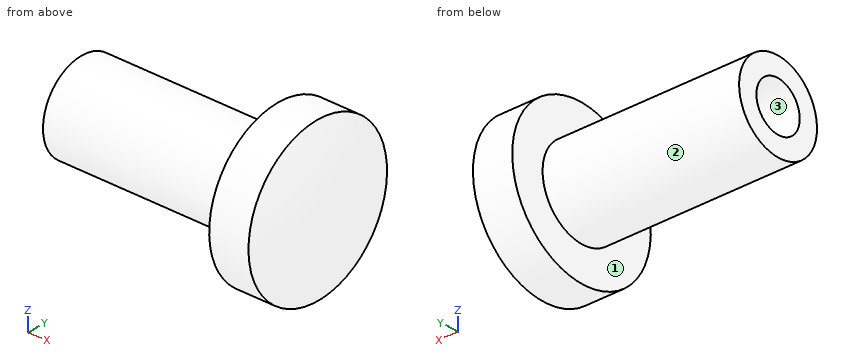
```python
from build123d import *

# Parameters (mm, degrees)
SKETCH2_R          = 1.25
CUT_EXTRUDE1_DEPTH = 11.25
SKETCH3_R          = 1.7
CUT_EXTRUDE2_DEPTH = 0.35


with BuildPart() as part:
    # Sketch1 → Revolve1 (revolve)
    with BuildSketch(Plane.XY, mode=Mode.PRIVATE) as revolve1_sk:
        with BuildLine():
            Line((0, 0), (0, 2.25))
            Line((0, 2.25), (10, 2.25))
            Line((10, 2.25), (10, 4))
            Line((10, 4), (12, 4))
            ThreePointArc((12, 4), (12.635153756, 2.044657673), (12.85, 0))
            Line((12.85, 0), (0, 0))
        make_face()
    revolve(revolve1_sk.sketch.rotate(Axis((0, 0, 0), (1, 0, 0)), 90), axis=Axis((0, 0, 0), (1, 0, 0)))

    # Sketch2 → Cut-Extrude1 (cut)
    with BuildSketch(Plane.ZY):
        Circle(SKETCH2_R)
    extrude(amount=-CUT_EXTRUDE1_DEPTH, mode=Mode.SUBTRACT)

    # Sketch3 → Cut-Extrude2 (cut)
    with BuildSketch(Plane.ZY.offset(-11.25)):
        Circle(SKETCH3_R)
    extrude(amount=-CUT_EXTRUDE2_DEPTH, mode=Mode.SUBTRACT)


solid = part.part
```
Here's how the part is built. I have some questions about the finished solid (model axes, mm). Face numbers are marked on the shaded views. Coordinates: 2 decimals unless noted, no trailing zeros. Order: outer loops, then holes, each group sorted by start corner. A loop starts at its lowest first (then second) coordinate and runs counter-clockwise, first axis right, second up.
1) I need wall thicknesses on line 1 (Y direction, x = 4.25, z = 0); line 2 (Y direction, x = 11.45, z = 0); line 3 (Z direction, x = 0.75, y = 0.25). Which ranges of each line are inside material? Lowest first, please.
2) Imagine slicing it at B-B on y = 0. List the corners of the cut face in (x, z) for me.
3) We'd pull the mould along Z, two halves only. Please class the marked faces 1, 2 and 3: +Z half, -Z half, draft (parallel to the pull), parting line (faces both ways), or undercut.
4) Will these pins go through, and if not, where does the flat tip stop? pin 1 (1 mm diameter, centred on y = 0.5, z = -0.5, fed in from -X); pin 2 (1 mm diameter, centred on y = 0.5, z = 0.5, fed in from +X); pin 3 (2 mm diameter, centred on x = 4, z = -0.5, fed in from +Y).
5) Imagine slicing it at A-A on x = 4.25. List the corners of the cut face in (y, z) for me.
6) Imagine slicing it at D-D on x = 10.5. List the corners of the cut face in (y, z) for me, and give its area (3 significant figures).
Response values:
1. line 1: y = -2.25 to -1.25, 1.25 to 2.25
1. line 2: y = -4 to -1.7, 1.7 to 4
1. line 3: z = -2.24 to -1.22, 1.22 to 2.24
2. outline: (0, -2.25) - (10, -2.25) - (10, -4) - (12, -4) arc R9.84 ccw to (12, 4) - (10, 4) - (10, 2.25) - (0, 2.25) - (0, 1.25) - (11.25, 1.25) - (11.25, 1.7) - (11.6, 1.7) - (11.6, -1.7) - (11.25, -1.7) - (11.25, -1.25) - (0, -1.25) - close
3. face 1: draft
3. face 2: parting line
3. face 3: undercut
4. pin 1: stops at x = 11.6
4. pin 2: stops at x = 12.85
4. pin 3: stops at y = 2.25
5. outline: circle Ø4.5 at (0, 0); hole circle Ø2.5 at (0, 0)
6. outline: circle Ø8 at (0, 0); hole circle Ø2.5 at (0, 0)
6. area: 45.4 mm2
